Geometry: final body of the model. Coordinates: model frame, mm. Give positions to 0.01 mm unless a question says otherwise; leave off trailing zeros. Loops run counter-clockwise (first coordinate to the right, second up) from the corner with the lowest first, then second, coordinate; pieces in that order, holes last.
from build123d import *

# Parameters (mm, degrees)
ESQUISSE1_R             = 61.5
BOSS_EXTRU_1_DEPTH      = 3
ESQUISSE3_W             = 30.466369815
ESQUISSE3_H             = 114.600421842
ENL_V_MAT_EXTRU_1_DEPTH = 4
D_GAGEMENT_M31_D        = 3.4
D_GAGEMENT_M3_51_D      = 3.9
ESQUISSE15_W            = 50
ESQUISSE15_H            = 21
ESQUISSE15_W_2          = 80
ESQUISSE15_H_2          = 16.662747472
ENL_V_MAT_EXTRU_2_DEPTH = 4


with BuildPart() as part:
    # Esquisse1 → Boss.-Extru.1 (new body)
    with BuildSketch(Plane(origin=(0, 0, 0), x_dir=(1, 0, 0), z_dir=(0, 1, 0))):
        Circle(ESQUISSE1_R)
    extrude(amount=BOSS_EXTRU_1_DEPTH)

    # Esquisse3 → Enlèv. mat.-Extru.1 (cut, through all)
    with BuildSketch(Plane(origin=(0, 3, 0), x_dir=(1, 0, 0), z_dir=(0, 1, 0))):
        with Locations((-55.233184908, -9.960159363)):
            Rectangle(ESQUISSE3_W, ESQUISSE3_H)
        with Locations((55.233184908, -9.960159363)):
            Rectangle(ESQUISSE3_W, ESQUISSE3_H)
    extrude(amount=-ENL_V_MAT_EXTRU_1_DEPTH, mode=Mode.SUBTRACT)

    # Dégagement M31 (through all)
    with Locations(Plane(origin=(0, 3, 0), x_dir=(1, 0, 0), z_dir=(0, 1, 0))):
        with Locations((-30, -8.5)):
            d_gagement_m31 = Hole(D_GAGEMENT_M31_D / 2)

    # Symétrie1: Dégagement M31 across plane
    add(d_gagement_m31.mirror(Plane.ZY), mode=Mode.SUBTRACT)

    # Dégagement M3.51 (through all)
    with Locations(Plane(origin=(0, 3, 0), x_dir=(1, 0, 0), z_dir=(0, 1, 0))):
        with Locations((-30, 42.5), (30, 42.5), (30, -42.5), (-30, -42.5)):
            Hole(D_GAGEMENT_M3_51_D / 2)

    # Esquisse15 → Enlèv. mat.-Extru.2 (cut, through all)
    with BuildSketch(Plane(origin=(0, 3, 0), x_dir=(1, 0, 0), z_dir=(0, 1, 0))):
        with Locations((0, 33)):
            Rectangle(ESQUISSE15_W, ESQUISSE15_H)
        with Locations((0, -55.045932494)):
            Rectangle(ESQUISSE15_W_2, ESQUISSE15_H_2)
        with Locations((0, -31)):
            Rectangle(ESQUISSE15_W, ESQUISSE15_H)
        with Locations((0, 1)):
            Rectangle(ESQUISSE15_W, ESQUISSE15_H)
    extrude(amount=-ENL_V_MAT_EXTRU_2_DEPTH, mode=Mode.SUBTRACT)


solid = part.part
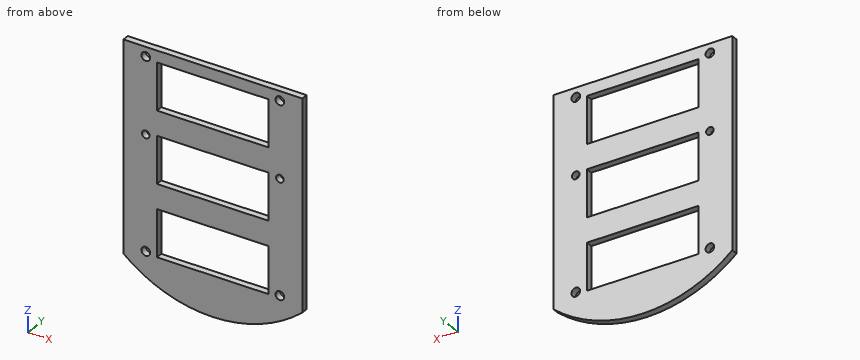
Item 1: Section query C-C on y = 1.45. Give the number of separate pieces and of enclosed holes in the cut face, plus the area to 3 significant figures.
Values follow:
separate pieces: 1
enclosed holes: 9
area: 5,070 mm2
Item 2: Ray query, probe 1 along X at (y, z) = (0.9, 42.5); probe 2 along X at (y, z) = (1.9, 37.5); probe 3 along Z at (x, y) = (-30, 1). Return the intervals inside material, ascending.
Values follow:
probe 1: x = -40 to -31.95, -28.05 to 28.05, 31.95 to 40
probe 2: x = -40 to -25, 25 to 40
probe 3: z = -53.69 to -44.45, -40.55 to 6.8, 10.2 to 40.55, 44.45 to 46.71
Item 3: Pin query (flat end, axial travel): pin 1 (5 mm diameter, centred on x = 30, z = 42.5, fed in from +Y); pin 2 (1.5 mm diameter, centred on x = 14.5, z = 7, fed in from +Y); pin 3 (1.5 mm diameter, centred on x = 2.5, y = 1.5, fed in from -Z); pin 4 (0.9 mm diameter, centred on x = 3.5, y = 1, fed in from -Z). Return the tip coordinate at first contact, or that it passes through.
Values follow:
pin 1: stops at y = 3
pin 2: passes through
pin 3: stops at z = -61.48
pin 4: stops at z = -61.42
Item 4: Section query D-D on x = -4.5. Return loops of the section in (y, z).
Values follow:
outline: (0, -61.34) - (3, -61.34) - (3, -43.5) - (0, -43.5) - close; (0, -22.5) - (3, -22.5) - (3, -11.5) - (0, -11.5) - close; (0, 9.5) - (3, 9.5) - (3, 20.5) - (0, 20.5) - close; (0, 41.5) - (3, 41.5) - (3, 46.71) - (0, 46.71) - close
Item 5: Section query B-B on x = -21.5. Return loops of the section in (y, z), plus the area to 3 significant figures.
Values follow:
outline: (0, -57.62) - (3, -57.62) - (3, -43.5) - (0, -43.5) - close; (0, -22.5) - (3, -22.5) - (3, -11.5) - (0, -11.5) - close; (0, 9.5) - (3, 9.5) - (3, 20.5) - (0, 20.5) - close; (0, 41.5) - (3, 41.5) - (3, 46.71) - (0, 46.71) - close
area: 124 mm2
Item 6: Section query A-A on z = 28. Return loops of the section in (x, y).
Values follow:
outline: (-40, 0) - (-25, 0) - (-25, 3) - (-40, 3) - close; (25, 0) - (40, 0) - (40, 3) - (25, 3) - close
